Job drawing, mm, ordinate dimensions from the low corner. One solid piece. Round coordinates to 2 decimals unless told otherwise and drop trailing zeros. Write each loop counter-clockwise with the first axis right and the second up, starting at its lowest first coordinate (ties: lowest second). Pieces come first, ordered by that corner, then holes.
1) Flat gauge pins, fed straight in: pin 1 (1.5 mm diameter, centred on y = 23, z = 5.5, fed in from +X); pin 2 (8 mm diameter, centred on x = 23.5, z = 16.5, fed in from -Y) (1 decimal); pin 3 (12 mm diameter, centred on x = 34.5, z = 10, fed in from +Y). Where does each tip first touch, or does it go through?
2) Saw through at B-B (z = 3.25). Write the cut outline in (x, y) (1 decimal), plus the area to 3 significant figures.
3) Wall check: probe 1 along X at (y, z) = (31.5, 12.75) (1 decimal); probe 2 along Y at (x, z) = (32.5, 16.5) (1 decimal); probe 3 along X at (y, z) = (33, 18.75) (1 decimal). Give the ranges that are in metal, low to high.
4) Saw through at A-A (z = 14.25). Write the cut outline in (x, y) (1 decimal).
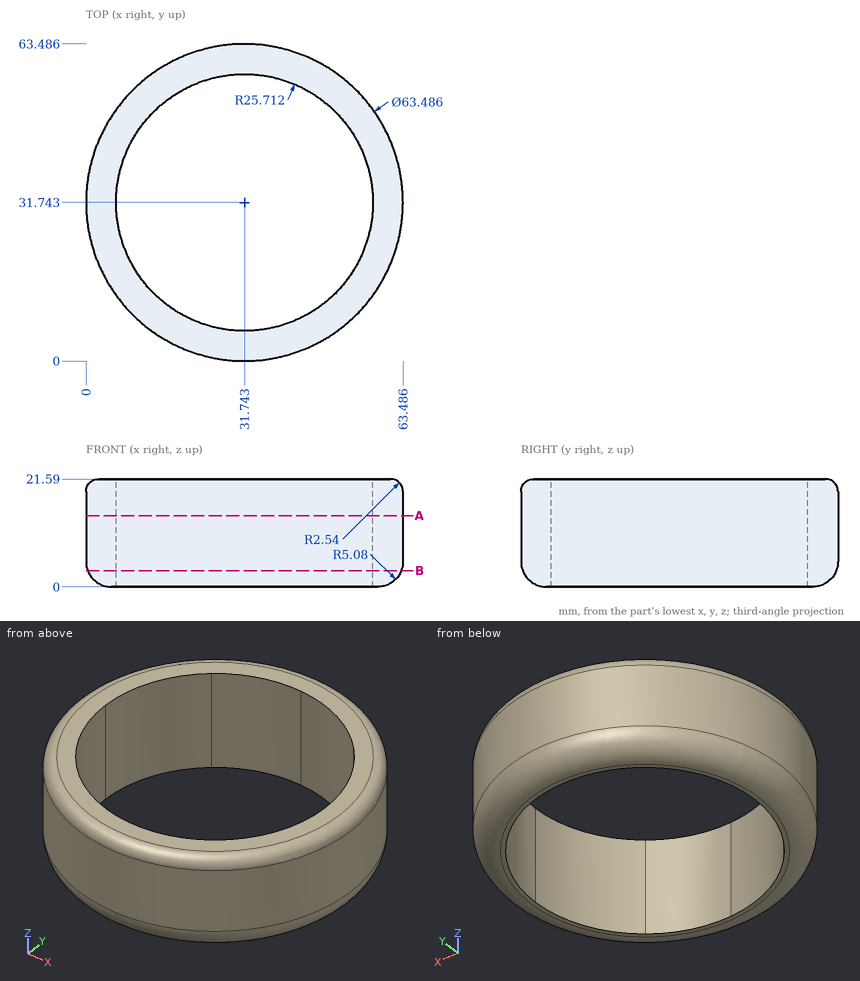
Evaluation:
1. pin 1: stops at x = 62.46
1. pin 2: stops at y = 0.3
1. pin 3: stops at y = 63.49
2. outline: circle Ø62.8 at (31.7, 31.7); hole (6, 31.7) arc R25.7 ccw to (13.5, 13.6) arc R25.7 ccw to (31.7, 6) arc R25.7 ccw to (47.6, 11.5) arc R25.7 ccw to (57.5, 31.7) arc R25.7 ccw to (50.2, 49.6) arc R25.7 ccw to (31.7, 57.5) arc R25.7 ccw to (15.4, 51.6) arc R25.7 ccw to start
2. area: 1,020 mm2
3. probe 1: x = 0 to 6, 57.5 to 63.5
3. probe 2: y = 0 to 6, 57.4 to 63.5
3. probe 3: x = 0 to 6.1, 57.4 to 63.5
4. outline: circle Ø63.5 at (31.7, 31.7); hole (6, 31.7) arc R25.7 ccw to (13.5, 13.6) arc R25.7 ccw to (31.7, 6) arc R25.7 ccw to (47.6, 11.5) arc R25.7 ccw to (57.5, 31.7) arc R25.7 ccw to (50.2, 49.6) arc R25.7 ccw to (31.7, 57.5) arc R25.7 ccw to (15.4, 51.6) arc R25.7 ccw to start
